```python
from build123d import *

# Parameters (mm, degrees)
F0_R     = 4
F0_W     = 3
F0_H     = 44
F0_R_2   = 1.5
F1_DEPTH = 3
F2_DEPTH = 18
F3_R     = 1.7
F4_DEPTH = 50
F5_DEPTH = 43


# Not quite as in the source:
# - a feature names something its author has since deleted; it is built from what else it names


with BuildPart() as f1:
    # F0 (on Top) → F1 (new body)
    with BuildSketch(Plane.XY):
        with BuildLine():
            Line((14, 22), (-22, 22))
            Line((-22, 22), (-22, -22))
            Line((-22, -22), (22, -22))
            Line((22, -22), (22, 18))
            ThreePointArc((22, 18), (18, 14), (14, 18))
            Line((14, 18), (14, 18.3849148452))
            Line((14, 18.3849148452), (14, 22))
        make_face()
        with Locations((0, -16)):
            Circle(F0_R, mode=Mode.SUBTRACT)
        with Locations((-23.5, 0)):
            Rectangle(F0_W, F0_H)
        Polygon((22, 18), (22, -22), (25, -22), (25, 22), (22, 22), align=None)
        with Locations((0, -16)):
            Circle(F0_R)
        with Locations((0, -16)):
            Circle(F0_R_2, mode=Mode.SUBTRACT)
    extrude(amount=F1_DEPTH)

    # F0 (on Top) → F2 (join)
    with BuildSketch(Plane.XY):
        with Locations((-23.5, 0)):
            Rectangle(F0_W, F0_H)
        Polygon((22, 18), (22, -22), (25, -22), (25, 22), (22, 22), align=None)
    extrude(amount=-F2_DEPTH)

    # F3 (on face) → F4 (cut, symmetric)
    with BuildSketch(Plane.YZ.offset(-22)):
        with Locations((-12, -12.4)):
            Circle(F3_R)
        with Locations((12, -12.4)):
            Circle(F3_R)
    extrude(amount=F4_DEPTH, both=True, mode=Mode.SUBTRACT)

    # F0 (on Top) → F5 (join)
    with BuildSketch(Plane.XY):
        with Locations((0, -16)):
            Circle(F0_R)
        with Locations((0, -16)):
            Circle(F0_R_2, mode=Mode.SUBTRACT)
    extrude(amount=F5_DEPTH)


solid = f1.part
```
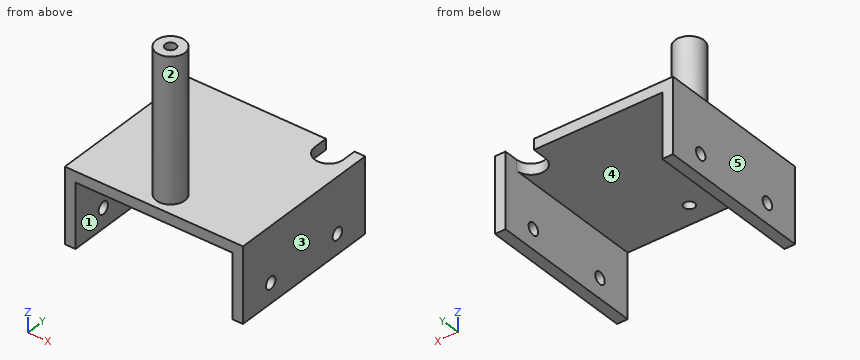
Model file for the job. Use its own axes, mm. Face numbers are marked on the shaded views. A direction names the side the tool comes from. Coordinates: 2 decimals unless noted, no trailing zeros. Order: outer loops, then holes, each group sorted by start corner. A loop starts at its lowest first (then second) coordinate and runs counter-clockwise, first axis right, second up. Notation, with made-up numbers: (-1, -29.75) -> (47, -29.75) arc R12 cw to (47, -6.75) -> close; hole circle Ø3 at (-18.75, -8.5). An arc over 180 degrees is marked (long way). Answer as a JSON object with one key per item and string values. Group by question number.
1) Drill centre lines: L1, parallel to X at y = -10, z = -5.5; L2, parallel to Y at x = 23, z = -12; L3, parallel to Z at x = -23.7, y = 12. Where is each one in solid material? Low to high.
2) Cut at C-C, the plane y = 12. Write the cut outline in (x, z).
3) Pull direction X, two halves, no side cores. Call the marked faces 3, 4 and 5: +X half, -X half, draft (parallel to the pull), parting line (faces both ways), or undercut.
4) Flat gauge pins, fed straight in: pin 1 (2 mm diameter, centred on x = 12.5, y = -5, fed in from -Z); pin 2 (3 mm diameter, centred on x = -1.5, z = 15.5, fed in from +Y); pin 3 (12 mm diameter, centred on x = -8.5, z = 32.5, fed in from -Y). Where does each tip first touch, or does it go through?
5) Cut at D-D, the plane y = -9.5. Write the cut outline in (x, z).
6) Cut at A-A, the plane y = -16. Write the cut outline in (x, z).
7) Cut at B-B, the plane z = -12.4. Write the cut outline in (x, y).
8) Which spindle directions (+Z, -Z, +X, -X, +Y, -Y) get a long thin tool onto all of the face, cutting with end or side? Do the marked faces 1 and 2. Say none if no direction does.
Check values:
{
 "1": {"L1": "x = -25 to -22, 22 to 25", "L2": "y = -22 to -13.65, -10.35 to 10.35, 13.65 to 22", "L3": "z = -18 to -14.1, -10.7 to 3"},
 "2": {"outline": "(-25, -18) -> (-22, -18) -> (-22, -14.1) -> (-25, -14.1) -> close; (-25, -10.7) -> (-22, -10.7) -> (-22, 0) -> (22, 0) -> (22, -10.7) -> (25, -10.7) -> (25, 3) -> (-25, 3) -> close; (22, -18) -> (25, -18) -> (25, -14.1) -> (22, -14.1) -> close"},
 "3": {"face 3": "+X half", "face 4": "undercut", "face 5": "-X half"},
 "4": {"pin 1": "stops at z = 0", "pin 2": "stops at y = -12", "pin 3": "stops at y = -19.12"},
 "5": {"outline": "(-25, -18) -> (-22, -18) -> (-22, 0) -> (22, 0) -> (22, -18) -> (25, -18) -> (25, 3) -> (-25, 3) -> close"},
 "6": {"outline": "(-25, -18) -> (-22, -18) -> (-22, 0) -> (-1.5, 0) -> (-1.5, 43) -> (-4, 43) -> (-4, 3) -> (-25, 3) -> close; (1.5, 0) -> (22, 0) -> (22, -18) -> (25, -18) -> (25, 3) -> (4, 3) -> (4, 43) -> (1.5, 43) -> close"},
 "7": {"outline": "(-25, -22) -> (-22, -22) -> (-22, -13.7) -> (-25, -13.7) -> close; (-25, -10.3) -> (-22, -10.3) -> (-22, 10.3) -> (-25, 10.3) -> close; (-25, 13.7) -> (-22, 13.7) -> (-22, 22) -> (-25, 22) -> close; (22, -22) -> (25, -22) -> (25, -13.7) -> (22, -13.7) -> close; (22, -10.3) -> (25, -10.3) -> (25, 10.3) -> (22, 10.3) -> close; (22, 13.7) -> (25, 13.7) -> (25, 22) -> (22, 22) -> close"},
 "8": {"face 1": "-Z, +Y, -Y", "face 2": "+Z"}
}
